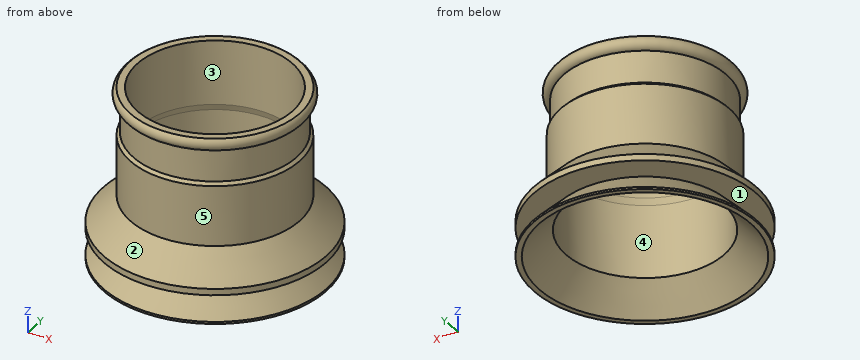
```python
from build123d import *


# Not quite as in the source:
# - a feature names something its author has since deleted; it is built from what else it names


with BuildPart() as f1:
    # F0 (on Front) → F1 (revolve)
    with BuildSketch(Plane.XZ):
        with BuildLine():
            Line((52, -12.5), (39.5, 0))
            Line((39.5, 0), (52, 0))
            Line((52, 0), (52, 3))
            Line((52, 3), (39.5, 3))
            Line((39.5, 3), (39.5, 15.5))
            Line((39.5, 15.5), (39.5, 43.6252272915))
            Line((39.5, 43.6252272915), (38.1252272915, 45))
            Line((38.1252272915, 45), (38.1252272915, 60))
            ThreePointArc((38.1252272915, 60), (40.9990174252, 62.4871708245), (39.5482522386, 66))
            Line((39.5482522386, 66), (36.1252272915, 66))
            Line((36.1252272915, 66), (36.1252272915, 36))
            Line((36.1252272915, 36), (37, 33))
            Line((37, 33), (37, -1.0355339059))
            Line((37, -1.0355339059), (49.4644660941, -13.5))
            Line((49.4644660941, -13.5), (52, -13.5))
            Line((52, -13.5), (52, -12.5))
        make_face()
        Polygon((39.5, 3), (52, 3), (39.5, 15.5), align=None)
    revolve(axis=Axis((0, 0, 34.5994567809), (0, 0, -1)))


solid = f1.part
```
The model under review builds one solid part; all positions refer to its coordinate system, in mm. Face numbers are marked on the shaded views. A direction names the side the tool comes from. Coordinates: 2 decimals unless noted, no trailing zeros.
1) To check wall thickness, follow probe 1 along X at (y, z) = (0, 50); probe 2 along X at (y, z) = (0, 22). State the ranges of each line that lie inside material, in increasing order.
2) Machinability: for the marked faces 4 and 5, which of the approach directions +Z, -Z, +X, -X, +Y, -Y give a long, thin tool a straight path to every point of the face, cutting with its end or side? Answer none if there is none.
3) The part is to be moulded in two halves that separate along Y. For the marked faces 1, 2 and 3, say which applies: pulls with the +Y half, pulls with the -Y half, needs draft (parallel to the pull), parting line crosses it, or undercut.
4) Clearance check with flat-ended pins moving along their axes: pin 1 Ø3 at (y, z) = (26, 14.5) entering from -X; pin 2 Ø10 at (y, z) = (36, -4) entering from -X; pin 3 Ø1 at (x, z) = (24.5, 35) entering from +Y. State where each tip first meets the part, or that it passes through.
Answer list:
1. probe 1: x = -38.13 to -36.13, 36.13 to 38.13
1. probe 2: x = -39.5 to -37, 37 to 39.5
2. face 4: -Z
2. face 5: none
3. face 1: needs draft
3. face 2: parting line crosses it
3. face 3: undercut
4. pin 1: stops at x = -33.31
4. pin 2: stops at x = -40.19
4. pin 3: stops at y = 31.37
